Work out the finished part from the listing and answer in its coordinate system (mm). A direction names the side the tool comes from. Round coordinates to 2 decimals unless told otherwise and drop trailing zeros. Order: outer loops, then holes, each group sorted by start corner. A loop starts at its lowest first (then second) coordinate and runs counter-clockwise, first axis right, second up. Notation, with made-up numbers: (9.25, 32.25) -> (45.25, 32.25) arc R20 cw to (45.25, 38.25) -> close; hole circle Ø7 at (59, 24.5). An arc over 180 degrees is marked (long way). Use a Markdown table: item, result. Add a question column.
Item 1: A tool of negligible diameter and unlimited length cuts with its end or side. For faces 4 (the flat face through (-16, -60, 7)), 5 (the flat face through (38, -51, 41)), 6 (the flat face through (-18, -60, 14)), 7 (the flat face through (-54, -51, 20)), 8 (the flat face through (-1, -23, 32)), from which of +Z, -Z, +X, -X, +Y, -Y can it reach the whole face along a straight path? Write none if from no direction.
Item 2: A cutting plane is placed at B-B, the plane y = -42. Determine the outline of the cut face in (x, z).
Item 3: Flat-ended cylindrical pins translate along their axes: P1, Ø4.5, axis at x = -18.5, y = -54.5, coming from the +Z side; P2, Ø1, axis at x = -38, y = -70.5, coming from the +Z side; P3, Ø1.5, axis at x = 18.5, y = -66.5, coming from the +Z side. Find the tip coordinate at first contact, or state that the pin passes through.
Item 4: A cutting plane is placed at D-D, the plane x = 5.5. Determine the outline of the cut face in (y, z), plus the area to 3 significant figures.
Item 5: For a pull along X with two mould halves and no side action, classify faces 1 (the cylindrical face through (48.1, -36.6, 9.9)), 2 (the flat face through (54, -51, 20)), 3 (the flat face through (-38, -51, 41)) as +X half, -X half, draft (parallel to the pull), parting line (faces both ways), or undercut.
Item 6: Find the intervals of material crossed by L1, parallel to Y at x = 56, z = 8; L2, parallel to X at y = -40, z = 13; L3, parallel to Y at x = 54, z = 13.25, in increasing order. Write a range as [from, to].
Item 7: A cutting plane is placed at A-A, the plane z = 26. Determine the outline of the cut face in (x, y).
Item 8: A cutting plane is placed at C-C, the plane z = 6. Determine the outline of the cut face in (x, y), plus the area to 3 significant figures.
from build123d import *

# Parameters (mm, degrees)
SKETCH1_R              = 20
BOSS_EXTRUDE1_DEPTH    = 32
BOSS_EXTRUDE3_DEPTH    = 20
SKETCH16_W             = 32
SKETCH16_H             = 56
BOSS_EXTRUDE4_DEPTH    = 20
F_16_0MM_DOWEL_HOLE3_D = 16
LPATTERN5_COUNT        = 2
LPATTERN5_PITCH        = 28
MIRROR5_COPY_1_D       = 16
SKETCH25_R             = 8
BOSS_EXTRUDE6_DEPTH    = 18
SKETCH26_W             = 14
SKETCH26_H             = 48
BOSS_EXTRUDE7_DEPTH    = 4


with BuildPart() as part:
    # Sketch1 → Boss-Extrude1 (new body)
    with BuildSketch(Plane.XY):
        with BuildLine():
            Line((-38, 0), (-38, -36))
            Line((-38, -36), (38, -36))
            Line((38, -36), (38, 0))
            ThreePointArc((38, 0), (0, 38), (-38, 0))
        make_face()
        Circle(SKETCH1_R, mode=Mode.SUBTRACT)
    extrude(amount=BOSS_EXTRUDE1_DEPTH)

    # Sketch15 → Boss-Extrude3 (add)
    with BuildSketch(Plane.XY):
        with BuildLine():
            Line((-70, -28), (-38, -28))
            Line((-38, -28), (-38, 0))
            ThreePointArc((-38, 0), (-48.739708375, -20.011761858), (-70, -28))
        make_face()
    boss_extrude3 = extrude(amount=BOSS_EXTRUDE3_DEPTH)

    # Sketch16 → Boss-Extrude4 (add)
    with BuildSketch(Plane.XY):
        with Locations((-54, -56)):
            Rectangle(SKETCH16_W, SKETCH16_H)
    boss_extrude4 = extrude(amount=BOSS_EXTRUDE4_DEPTH)

    # Ø16.0mm Dowel Hole3 (through all)
    with Locations(Plane.XY.offset(20)):
        with Locations((-54, -42)):
            f_16_0mm_dowel_hole3 = Hole(F_16_0MM_DOWEL_HOLE3_D / 2)

    # LPattern5: Ø16.0mm Dowel Hole3 ×2
    with Locations(*[(0, -i * LPATTERN5_PITCH, 0) for i in range(1, LPATTERN5_COUNT)]):
        add(f_16_0mm_dowel_hole3, mode=Mode.SUBTRACT)

    # Mirror5: Boss-Extrude4, Boss-Extrude3, Ø16.0mm Dowel Hole3 across plane
    add(boss_extrude4.mirror(Plane(origin=(0, 0, 0), x_dir=(0, 0, 1), z_dir=(1, 0, 0))))
    add(boss_extrude3.mirror(Plane(origin=(0, 0, 0), x_dir=(0, 0, 1), z_dir=(1, 0, 0))))
    add(f_16_0mm_dowel_hole3.mirror(Plane(origin=(0, 0, 0), x_dir=(0, 0, 1), z_dir=(1, 0, 0))), mode=Mode.SUBTRACT)

    # Mirror5 copy 1 (through all)
    with Locations(Plane(origin=(0, -28, 20), x_dir=(-1, 0, 0), z_dir=(0, 0, 1))):
        with Locations((-54, 42)):
            Hole(MIRROR5_COPY_1_D / 2)

    # Sketch25 → Boss-Extrude6 (add)
    with BuildSketch(Plane(origin=(-38, 0, 0), x_dir=(0, 0, -1), z_dir=(1, 0, 0))):
        with BuildLine():
            Line((0, -84), (-60, -84))
            ThreePointArc((-60, -84), (-75.567317873, -71.695756248), (-67.191626537, -53.707326781))
            Line((-67.191626537, -53.707326781), (-32, -36))
            Line((-32, -36), (0, -36))
            Line((0, -36), (0, -84))
        make_face()
        with Locations(Location((-60, -68, 0), (0, 0, 90))):  # turned: the seam where the file's is
            Circle(SKETCH25_R, mode=Mode.SUBTRACT)
    boss_extrude6 = extrude(amount=BOSS_EXTRUDE6_DEPTH)

    # Sketch26 → Boss-Extrude7 (add)
    with BuildSketch(Plane(origin=(-20, 0, 0), x_dir=(0, 0, -1), z_dir=(1, 0, 0))):
        with Locations((-7, -60)):
            Rectangle(SKETCH26_W, SKETCH26_H)
    boss_extrude7 = extrude(amount=BOSS_EXTRUDE7_DEPTH)

    # Mirror6: Boss-Extrude6, Boss-Extrude7 across plane
    add(boss_extrude6.mirror(Plane(origin=(0, 0, 0), x_dir=(0, 0, 1), z_dir=(1, 0, 0))))
    add(boss_extrude7.mirror(Plane(origin=(0, 0, 0), x_dir=(0, 0, 1), z_dir=(1, 0, 0))))


solid = part.part
Reported:
| question | item | result |
|---|---|---|
| 1 | face 4 | +Z, -Z, -Y |
| 1 | face 5 | +Z, +X, +Y, -Y |
| 1 | face 6 | +Z, -Y |
| 1 | face 7 | +Z, -X, +Y, -Y |
| 1 | face 8 | +Z, +X, -X, +Y |
| 2 | outline | (-70, 0) -> (-62, 0) -> (-62, 20) -> (-70, 20) -> close; (-46, 0) -> (-16, 0) -> (-16, 14) -> (-20, 14) -> (-20, 43.92) -> (-38, 43.92) -> (-38, 20) -> (-46, 20) -> close; (16, 0) -> (46, 0) -> (46, 20) -> (38, 20) -> (38, 43.92) -> (20, 43.92) -> (20, 14) -> (16, 14) -> close; (62, 0) -> (70, 0) -> (70, 20) -> (62, 20) -> close |
| 3 | P1 | z = 70.78 |
| 3 | P2 | z = 75.87 |
| 3 | P3 | z = 14 |
| 4 | outline | (-36, 0) -> (-19.23, 0) -> (-19.23, 32) -> (-36, 32) -> close; (19.23, 0) -> (37.6, 0) -> (37.6, 32) -> (19.23, 32) -> close |
| 4 | area | 1,120 mm² |
| 5 | face 1 | undercut |
| 5 | face 2 | draft |
| 5 | face 3 | -X half |
| 6 | L1 | [-84, -77.75], [-62.25, -49.75], [-34.25, -24.81] |
| 6 | L2 | [-70, -61.75], [-46.25, -16], [16, 46.25], [61.75, 70] |
| 6 | L3 | [-84, -78], [-62, -50], [-34, -23.76] |
| 7 | outline | (-38, -84) -> (-20, -84) -> (-20, -36) -> (20, -36) -> (20, -84) -> (38, -84) -> (38, 0) arc R38 ccw to (-38, 0) -> close; hole circle Ø40 at (0, 0) |
| 8 | outline | (-70, -84) -> (-16, -84) -> (-16, -36) -> (16, -36) -> (16, -84) -> (70, -84) -> (70, -28) arc R32.29 cw to (38, 0) arc R38 ccw to (-38, 0) arc R32.29 cw to (-70, -28) -> close; hole circle Ø16 at (-54, -70); hole circle Ø16 at (-54, -42); hole circle Ø40 at (0, 0); hole circle Ø16 at (54, -70); hole circle Ø16 at (54, -42) |
| 8 | area | 9,070 mm² |
